Autodesk Inventor part; units mm, degrees
ref_plane "YZ Plane" through (0, 0, 0) normal (1, 0, 0) x (0, 1, 0)
ref_plane "XZ Plane" through (0, 0, 0) normal (0, 1, 0) x (-1, 0, 0)
ref_plane "XY Plane" through (0, 0, 0) normal (0, 0, 1) x (1, 0, 0)
sketch "スケッチ1" plane through (0, 0, 0) normal (0, 0, 1) x (1, 0, 0)
  circle A0 centre (0, 0) radius 11.05
  line L0 (30, 30) -> (-30, 30) construction
  line L1 (-30, 30) -> (-30, -30) construction
  line L2 (-30, -30) -> (30, -30) construction
  line L3 (30, -30) -> (30, 30) construction
  line L4 (30, 30) -> (-30, -30) construction
  line L5 (-30, 30) -> (30, -30) construction
  circle A1 centre (-30, 30) radius 1.6
  circle A2 centre (30, 30) radius 1.6
  circle A3 centre (30, -30) radius 1.6
  circle A4 centre (-30, -30) radius 1.6
  circle A5 centre (-30, 0) radius 1.6
  circle A6 centre (30, 0) radius 1.6
  circle A7 centre (0, 300) radius 10 construction
  line L6 (0, 300) -> (82.4797, 11.5609) construction
  line L7 (0, 300) -> (132.9888, 31.0874) construction
  arc A8 (0, 0) -> (244.9763, 126.8336) centre (0, 300) ccw construction
  line L8 (106.8619, 8.1323) -> (101.3633, 27.3615) construction
  circle A9 centre (82.4797, 11.5609) radius 11.05
  line L9 (96.2103, 36.2888) -> (57.7518, 25.2915) construction
  line L10 (101.3633, 27.3615) -> (58.0974, 14.9896) construction
  line L11 (58.0974, 14.9896) -> (106.8619, 8.1323) construction
  line L12 (101.3633, 27.3615) -> (63.5961, -4.2397) construction
  line L13 (63.5961, -4.2397) -> (106.8619, 8.1323) construction
  line L14 (96.2103, 36.2888) -> (68.7491, -13.167) construction
  circle A10 centre (82.4797, 11.5609) radius 23.5 construction
  line L15 (68.7491, -13.167) -> (107.2076, -2.1697) construction
  circle A11 centre (63.5961, -4.2397) radius 1.6
  line L16 (58.0974, 14.9896) -> (63.5961, -4.2397) construction
  line L17 (57.7518, 25.2915) -> (68.7491, -13.167) construction
  circle A12 centre (101.3633, 27.3615) radius 1.6
  circle A13 centre (101.3633, 27.3615) radius 5 construction
  circle A14 centre (107.2076, -2.1697) radius 1.6
  arc A15 (111.2054, -2.0356) -> (105.4181, -5.7471) centre (107.2076, -2.1697) ccw construction
  circle A16 centre (68.7491, -13.167) radius 1.6
  circle A17 centre (57.7518, 25.2915) radius 1.6
  circle A18 centre (106.8619, 8.1323) radius 1.6
  line L18 (107.2076, -2.1697) -> (96.2103, 36.2888) construction
  circle A19 centre (58.0974, 14.9896) radius 1.6
  circle A20 centre (96.2103, 36.2888) radius 1.6
  circle A21 centre (58.0974, 14.9896) radius 5 construction
  line L19 (57.7518, 25.2915) -> (107.2076, -2.1697) construction
  line L20 (37.5, 43.7095) -> (22.5, 43.7095) construction
  line L21 (22.5, 43.7095) -> (22.5, -43.7095) construction
  line L22 (22.5, -43.7095) -> (37.5, -43.7095) construction
  line L23 (37.5, -43.7095) -> (37.5, 43.7095) construction
  line L24 (37.5, 43.7095) -> (22.5, -43.7095) construction
  line L25 (22.5, 43.7095) -> (37.5, -43.7095) construction
  circle A22 centre (132.9888, 31.0874) radius 23 construction
  arc A23 (-30, 35) -> (-35, 30) centre (-30, 30) ccw
  arc A24 (-35, -30) -> (-30, -35) centre (-30, -30) ccw
  arc A25 (30, -35) -> (31.7527, -34.6827) centre (30, -30) ccw
  arc A26 (100.5407, 38.7884) -> (95.7358, 41.2663) centre (96.2103, 36.2888) ccw construction
  line L26 (108.5253, -5.9475) -> (31.7527, -34.6827)
  line L27 (30, -35) -> (-30, -35)
  line L28 (-35, -30) -> (-35, 30)
  line L29 (-30, 35) -> (30, 35)
  line L30 (30, 35) -> (94.8682, 41.1836)
  circle A27 centre (0, 0) radius 55 construction
  line L31 (142.0504, 57.8808) -> (106.1954, 40.149) construction
  line L32 (106.1954, 40.149) -> (123.9272, 4.294) construction
  line L33 (123.9272, 4.294) -> (159.7822, 22.0258) construction
  line L34 (159.7822, 22.0258) -> (142.0504, 57.8808) construction
  line L35 (142.0504, 57.8808) -> (123.9272, 4.294) construction
  line L36 (106.1954, 40.149) -> (159.7822, 22.0258) construction
  circle A28 centre (106.1954, 40.149) radius 1.6
  circle A29 centre (142.0504, 57.8808) radius 1.6
  circle A30 centre (159.7822, 22.0258) radius 1.6
  circle A31 centre (123.9272, 4.294) radius 1.6
  circle A32 centre (132.9888, 31.0874) radius 10
  circle A33 centre (120.674, 35.2523) radius 1.6
  circle A34 centre (137.1537, 43.4022) radius 1.6
  circle A35 centre (145.3036, 26.9225) radius 1.6
  circle A36 centre (128.8239, 18.7726) radius 1.6
  circle A37 centre (132.9888, 31.0874) radius 13 construction
  circle A38 centre (124.1229, 49.0149) radius 1.6
  circle A39 centre (141.8547, 13.1599) radius 1.6
  circle A40 centre (106.1954, 40.149) radius 5 construction
  arc A41 (126.1437, -0.1879) -> (125.4672, -0.463) centre (123.9272, 4.294) ccw construction
  line L37 (101.7135, 37.9325) -> (119.4454, 2.0775) construction
  arc A42 (146.5323, 60.0973) -> (139.9198, 62.4042) centre (142.0504, 57.8808) ccw
  arc A43 (161.9987, 17.544) -> (164.2641, 24.2423) centre (159.7822, 22.0258) ccw
  line L38 (139.9198, 62.4042) -> (94.8682, 41.1836)
  line L39 (146.5323, 60.0973) -> (164.2641, 24.2423)
  line L40 (161.9987, 17.544) -> (126.1437, -0.1879)
  line L41 (108.5253, -5.9475) -> (125.4672, -0.463)
  arc A44 (125.4672, -0.463) -> (126.1437, -0.1879) centre (123.9272, 4.294) ccw
  circle A45 centre (115.0613, 22.2215) radius 1.6
  circle A46 centre (150.9163, 39.9533) radius 1.6
  point P0 (82.4797, 11.5609)
  dimension "d59" = 10
  dimension "d0" = 22.1
  dimension "d1" = 60
  dimension "d2" = 60
  dimension "d3" = 3.2
  dimension "d5" = 3.2
  dimension "d6" = 3.2
  dimension "d8" = 3.2
  dimension "d9" = 3.2
  dimension "d10" = 3.2
  dimension "d11" = 20
  dimension "d13" = 300
  dimension "d14" = 47
  dimension "d15" = 22.1
  dimension "d16" = 20
  dimension "d17" = 45
  dimension "d18" = 40
  dimension "d19" = 40
  dimension "d20" = 3.2
  dimension "d21" = 3.2
  dimension "d22" = 3.2
  dimension "d23" = 3.2
  dimension "d24" = 3.2
  dimension "d25" = 3.2
  dimension "d26" = 3.2
  dimension "d27" = 3.2
  dimension "d28" = 10
  dimension "d30" = 8
  dimension "d31" = 10
  dimension "d32" = 15
  dimension "d33" = 46
  dimension "d35" = 5
  dimension "d38" = 5
  dimension "d39" = 5
  dimension "d40" = 5
  dimension "d41" = 5
  dimension "d44" = 110
  dimension "d45" = 40
  dimension "d46" = 40
  dimension "d47" = 3.2
  dimension "d48" = 3.2
  dimension "d49" = 3.2
  dimension "d50" = 3.2
  dimension "d51" = 20
  dimension "d52" = 3.2
  dimension "d53" = 3.2
  dimension "d54" = 3.2
  dimension "d55" = 3.2
  dimension "d56" = 13
  dimension "d57" = 3.2
  dimension "d58" = 3.2
  dimension "d60" = 10
  dimension "d61" = 5
  dimension "d62" = 5
  dimension "d65" = 3.2
  dimension "d66" = 3.2
extrude "押し出し2" add sketch "スケッチ1" along normal blind 3
properties part number "関節3_側板左"
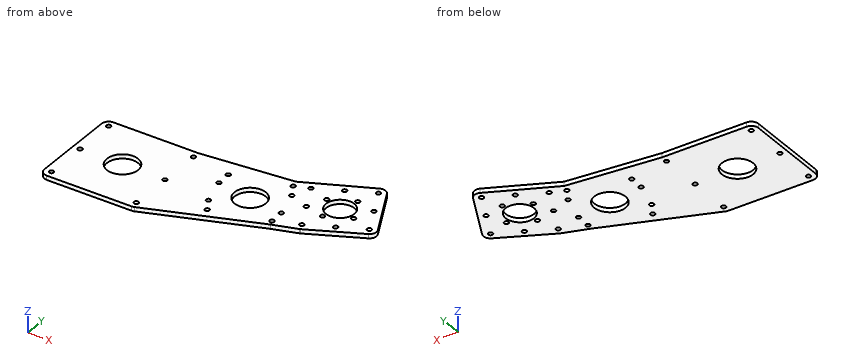
Design review of the part built by this model. Coordinates are the model's own, in mm. Coordinates: 2 decimals unless noted, no trailing zeros. Order: outer loops, then holes, each group sorted by start corner. A loop starts at its lowest first (then second) coordinate and runs counter-clockwise, first axis right, second up. Notation, with made-up numbers: M 9.5,-28 L 51.5,-28 A17 ccw 51.5,-10 Z; hole C 1.25,-9.5 d10. An arc over 180 degrees is marked long. Answer as a JSON object with one key per item and string values. Group by question number.
1) For pin 1 (1.5 mm diameter, centred on x = 1.5, z = 1, fed in from +Y); pin 2 (2.5 mm diameter, centred on x = 68.75, y = -13.17, fed in from +Z), all flat-tipped, find the tip position at first contact; note any pin that passes through.
2) Add section D-D, the plane x = 39. Write out the cut boundary in (y, z), then the cut area to 3 significant figures.
3) Add section B-B, the plane y = -18. Write out the cut boundary in (x, z).
4) Add section A-A, the plane x = 0. Write out the cut boundary in (y, z).
5) Wall thickness on L1, parallel to Y at x = 0, z = 1.15; L2, parallel to Y at x = 30, z = 1.85; L3, parallel to X at y = 29.5, z = 1.7: over which ranges is each line inside the solid? List them lowest first.
6) Add section C-C, the plane z = 2.2. Count the separate pieces of the cut face and the enclosed holes in it, then the cut area to 3 significant figures.
Computed values:
{
 "1": {"pin 1": "stops at y = 35", "pin 2": "passes through"},
 "2": {"outline": "M -31.97,0 L 35.86,0 L 35.86,3 L -31.97,3 Z", "area": "203 mm^2"},
 "3": {"outline": "M -35,0 L 76.32,0 L 76.32,3 L -35,3 Z"},
 "4": {"outline": "M -35,0 L -11.05,0 L -11.05,3 L -35,3 Z; M 11.05,0 L 35,0 L 35,3 L 11.05,3 Z"},
 "5": {"L1": "y = -35 to -11.05, 11.05 to 35", "L2": "y = -35 to -31.6, -28.4 to -1.6, 1.6 to 28.4, 31.6 to 35", "L3": "x = -35 to -31.52, -28.48 to 28.48, 31.52 to 123.12, 142.86 to 161.66"},
 "6": {"separate pieces": "1", "enclosed holes": "29", "area": "10,500 mm^2"}
}
